For this review, take the finished solid that the model builds, in its own axes (mm). A direction names the side the tool comes from. Give positions to 0.01 mm unless a question says otherwise; leave off trailing zeros. Loops run counter-clockwise (first coordinate to the right, second up) from the corner with the lowest first, then second, coordinate; pieces in that order, holes last. Notation, with made-up numbers: (49.25, 30.5) - (71.25, 30.5) arc R29 cw to (71.25, 54.5) - close; hole circle Ø1 at (84, 2). An arc over 180 degrees is marked (long way). Use CSV: the item, a comma, the result in double quotes. Start each with the question number.
1. Take a section at C-C on z = 3.55. Give the boundary of the cut face in (x, y).
2. Take a section at D-D on z = 1.05. Give the boundary of the cut face in (x, y), plus the area to 3 significant figures.
3. Take a section at B-B on x = 0. Give the boundary of the cut face in (y, z).
4. Take a section at A-A on y = 0. Give the boundary of the cut face in (x, z).
5. For faces 1 (the cylindrical face through (-2.38, -10.74, 1.24)), 2 (the cylindrical face through (3.558, 2.038, 3.976)), list the 3-axis set-ups (+Z, -Z, +X, -X, +Y, -Y) from which the entire face can be reached by the end or side of a thin tool; tool diameter is ignored.
6. Mouldability with a two-part tool opening along X and no side actions: class faces 3 (the cylindrical face through (3.544, -2.062, 3.976)), 4 (the cylindrical face through (0, -4.1, 4)), 5 (the cylindrical face through (-3.5, 0, 4)) as pulls with the +X half, pulls with the -X half, needs draft (parallel to the pull), parting line crosses it, or undercut.
7. For pin 1 (3 mm diameter, centred on x = -7, z = 1.5, fed in from -Y), flat-tipped, find the tip position at first contact; note if it passes through.
8. Wall thickness on line 1 (Z direction, x = 9, y = 3); line 2 (Z direction, x = 1.5, y = 3.5); line 3 (Y direction, x = -3.5, z = 1.85): over which ranges is each line inside the solid? List them lowest first.
```python
from build123d import *

# Parameters (mm, degrees)
SKETCH_R           = 11
PAD_DEPTH          = 2
CHAMFER_SIZE       = 0.5
SKETCH001_R        = 5
PAD001_DEPTH       = 0.3
SKETCH002_R        = 3.5
PAD002_DEPTH       = 3.4
SKETCH003_R        = 0.6
PAD003_DEPTH       = 3.4
POLARPATTERN_COUNT = 6


with BuildPart() as part:
    # Sketch → Pad (new body)
    with BuildSketch(Plane.XY):
        Circle(SKETCH_R)
    extrude(amount=PAD_DEPTH)

    # Chamfer
    chamfer_edges = [part.edges().sort_by_distance(p)[0] for p in [
        (-11, 0, 0),
    ]]
    chamfer(chamfer_edges, length=CHAMFER_SIZE)

    # Sketch001 → Pad001 (new body)
    with BuildSketch(Plane.XY.offset(2)):
        Circle(SKETCH001_R)
    extrude(amount=PAD001_DEPTH)

    # Sketch002 → Pad002 (new body)
    with BuildSketch(Plane.XY.offset(2.3)):
        Circle(SKETCH002_R)
    extrude(amount=PAD002_DEPTH)

    # Sketch003 → Pad003 (new body)
    with BuildSketch(Plane.XY.offset(2.3)):
        with Locations((0, 3.5)):
            Circle(SKETCH003_R)
    pad003 = extrude(amount=PAD003_DEPTH)

    # PolarPattern: Pad003 ×6 about axis
    polarpattern_axis = Axis((0, 0, 2.3), (0, 0, 1))
    for i in range(1, POLARPATTERN_COUNT):
        add(pad003.rotate(polarpattern_axis, i * 360 / POLARPATTERN_COUNT))


solid = part.part
```
Check result:
1,outline,"(-3.29, -1.21) arc R0.6 ccw (long way) to (-2.69, -2.24) arc R3.5 ccw to (-0.6, -3.45) arc R0.6 ccw (long way) to (0.6, -3.45) arc R3.5 ccw to (2.69, -2.24) arc R0.6 ccw (long way) to (3.29, -1.21) arc R3.5 ccw to (3.29, 1.21) arc R0.6 ccw (long way) to (2.69, 2.24) arc R3.5 ccw to (0.6, 3.45) arc R0.6 ccw (long way) to (-0.6, 3.45) arc R3.5 ccw to (-2.69, 2.24) arc R0.6 ccw (long way) to (-3.29, 1.21) arc R3.5 ccw to start"
2,outline,"circle Ø22 at (0, 0)"
2,area,"380 mm²"
3,outline,"(-11, 0.5) - (-10.5, 0) - (10.5, 0) - (11, 0.5) - (11, 2) - (5, 2) - (5, 2.3) - (4.1, 2.3) - (4.1, 5.7) - (-4.1, 5.7) - (-4.1, 2.3) - (-5, 2.3) - (-5, 2) - (-11, 2) - close"
4,outline,"(-11, 0.5) - (-10.5, 0) - (10.5, 0) - (11, 0.5) - (11, 2) - (5, 2) - (5, 2.3) - (3.5, 2.3) - (3.5, 5.7) - (-3.5, 5.7) - (-3.5, 2.3) - (-5, 2.3) - (-5, 2) - (-11, 2) - close"
5,face 1,"+Z, -Z"
5,face 2,"+Z"
6,face 3,"undercut"
6,face 4,"parting line crosses it"
6,face 5,"pulls with the -X half"
7,pin 1,"stops at y = -9.53"
8,line 1,"z = 0 to 2"
8,line 2,"z = 0 to 2.3"
8,line 3,"y = -10.43 to 10.43"
